```python
from build123d import *

# Parameters (mm, degrees)
SKETCH_1_W                       = 1.5
SKETCH_1_H                       = 210
SM_BASE_FLANGE_1_DEPTH           = 198.66
SKETCH_6_R                       = 2.75
CUT_EXTRUDE_1_DEPTH              = 10
SM_EDGE_FLANGE_1_STRIP_W         = 7.4732
SM_EDGE_FLANGE_1_STRIP_H         = 1.5
SM_EDGE_FLANGE_1_STRIP_CUT_DEPTH = 210
SM_EDGE_FLANGE_1_DEPTH           = 210


# Sheet-metal steps are written as plain solids
with BuildPart() as part:
    # Sketch 1 → 基体-法兰1 (new body)
    with BuildSketch(Plane.XY):
        with Locations((0.75, 105)):
            Rectangle(SKETCH_1_W, SKETCH_1_H)
    extrude(amount=SM_BASE_FLANGE_1_DEPTH)

    # 草图6 → 切除-拉伸1 (cut)
    with BuildSketch(Plane(origin=(1.5, 0, 0), x_dir=(0, 0, -1), z_dir=(1, 0, 0))):
        with Locations((-93.91, 55)):
            Circle(SKETCH_6_R)
        with Locations((-93.91, 155)):
            Circle(SKETCH_6_R)
        with Locations((-93.91, 105)):
            Circle(SKETCH_6_R)
    extrude(amount=-CUT_EXTRUDE_1_DEPTH, mode=Mode.SUBTRACT)

    # 边线-法兰1 strip (across the edge) → 边线-法兰1 strip cut (cut)
    with BuildSketch(Plane(origin=(0, 0, 198.66), x_dir=(0, 0, -1), z_dir=(0, 1, 0))):
        with Locations((-1.5, -0.75)):
            Rectangle(SM_EDGE_FLANGE_1_STRIP_W, SM_EDGE_FLANGE_1_STRIP_H)
    extrude(amount=SM_EDGE_FLANGE_1_STRIP_CUT_DEPTH, mode=Mode.SUBTRACT)

    # 边线-法兰1 section (across the edge) → 边线-法兰1 (add)
    with BuildSketch(Plane(origin=(0, 0, 198.66), x_dir=(0, 0, -1), z_dir=(0, 1, 0))):
        with BuildLine():
            Line((0, 0.7366), (0, 13.5))
            Line((0, 13.5), (1.5, 13.5))
            Line((1.5, 13.5), (1.5, 0.7366))
            ThreePointArc((1.5, 0.7366), (1.715745145, 0.215745145), (2.2366, 0))
            Line((2.2366, 0), (2.2366, -1.5))
            ThreePointArc((2.2366, -1.5), (0.655084973, -0.844915027), (0, 0.7366))
        make_face()
    extrude(amount=SM_EDGE_FLANGE_1_DEPTH)


solid = part.part
```
Verification items for the finished model (mm, model axes). A direction names the side the tool comes from. Round coordinates to 2 decimals unless told otherwise and drop trailing zeros. Write each loop counter-clockwise with the first axis right and the second up, starting at its lowest first coordinate (ties: lowest second). Pieces come first, ordered by that corner, then holes. Notation, with made-up numbers: (37.25, 19.5) -> (55.25, 19.5) arc R20 ccw to (55.25, 58.5) -> close; hole circle Ø11 at (23, -33.5). An arc over 180 degrees is marked (long way). Write each question's results on one line, items separated by ' | '.
Q1. Draft check along Y on faces 1 (the face through (0, 104, 97)), 2 (the face through (0.8, 57.3, 92.4)), 3 (the face through (1, 0, 99)). Enter one of: released by +Y, released by -Y, zero draft, split by the parting line, or undercut.
Derived:
face 1: zero draft | face 2: undercut | face 3: released by -Y
Q2. Sectioned sample at A-A, the plane z = 93.91. Record the boundary of the cut face in (x, y), and give its area (3 significant figures).
Derived:
outline: (0, 0) -> (1.5, 0) -> (1.5, 52.25) -> (0, 52.25) -> close; (0, 57.75) -> (1.5, 57.75) -> (1.5, 102.25) -> (0, 102.25) -> close; (0, 107.75) -> (1.5, 107.75) -> (1.5, 152.25) -> (0, 152.25) -> close; (0, 157.75) -> (1.5, 157.75) -> (1.5, 210) -> (0, 210) -> close | area: 290 mm²
Q3. Sectioned sample at D-D, the plane x = -5. Record the boundary of the cut face in (y, z), and give its area (3 significant figures).
Derived:
outline: (0, 197.16) -> (210, 197.16) -> (210, 198.66) -> (0, 198.66) -> close | area: 315 mm²
Q4. Access from +Z, -Z, +X, -X, +Y, -Y to the whole of each face (thin tool, end or side, straight path). Record for faces 4 (the face through (-7, 104, 197.16)), 5 (the face through (0.76, 102.56, 92.64)).
Derived:
face 4: -Z, -X, +Y, -Y | face 5: +X, -X
Q5. Sectioned sample at B-B, the plane y = 55. Record the boundary of the cut face in (x, z).
Derived:
outline: (-13.5, 197.16) -> (-0.74, 197.16) arc R0.74 cw to (0, 196.42) -> (0, 96.66) -> (1.5, 96.66) -> (1.5, 196.42) arc R2.24 ccw to (-0.74, 198.66) -> (-13.5, 198.66) -> close; (0, 0) -> (1.5, 0) -> (1.5, 91.16) -> (0, 91.16) -> close
Q6. Sectioned sample at C-C, the plane y = 178.5. Record the boundary of the cut face in (x, z), and give its area (3 significant figures).
Derived:
outline: (-13.5, 197.16) -> (-0.74, 197.16) arc R0.74 cw to (0, 196.42) -> (0, 0) -> (1.5, 0) -> (1.5, 196.42) arc R2.24 ccw to (-0.74, 198.66) -> (-13.5, 198.66) -> close | area: 317 mm²
Q7. Thickness scan on probe 1 along Y at (x, z) = (0.4, 93.91); probe 2 along Z at (x, y) = (-12.25, 190.5); probe 3 along X at (y, z) = (12.5, 133.5). Record the ranges inside material, lowest first.
Derived:
probe 1: y = 0 to 52.25, 57.75 to 102.25, 107.75 to 152.25, 157.75 to 210 | probe 2: z = 197.16 to 198.66 | probe 3: x = 0 to 1.5
Q8. Go/stop test with flat-tipped pins: pin 1 Ø4 at (x, z) = (-3.5, 145) entering from +Y; pin 2 Ø4 at (x, y) = (-7, 90) entering from -Z; pin 3 Ø5 at (y, z) = (139, 169) entering from -X. Record where each tip stops, or that it passes through.
Derived:
pin 1: passes through | pin 2: stops at z = 197.16 | pin 3: stops at x = 0
